The listing builds one solid part. Answer for the finished solid, in the listing's coordinates (mm). Face numbers are marked on the shaded views. A direction names the side the tool comes from. Give positions to 0.01 mm unless a question says otherwise; leave off trailing zeros. Loops run counter-clockwise (first coordinate to the right, second up) from the corner with the lowest first, then second, coordinate; pieces in that order, holes last. Notation, with made-up numbers: (44, 53) - (55, 53) arc R13 ccw to (55, 66) - close; hole circle Ø8 at (-26, 82). An arc over 180 degrees is marked (long way). Write item = value, one per line. Start each with the question number.
1) The part is cut by section D-D on z = 2.4. Write down the section's boundary in (x, y).
2) Flat-ended cylindrical pins translate along their axes: P1, Ø5.5, axis at x = 0, y = 0, coming from the +Z side; P2, Ø1.5, axis at x = -6.5, z = 2, coming from the +Y side. Find the tip coordinate at first contact, or state that the pin passes through.
3) The mould has two halves that part along Y. Classify the marked faces 4, 5, 6 and 7: +Y half, -Y half, draft (parallel to the pull), parting line (faces both ways), or undercut.
4) Consider probe 1 along Y at (x, z) = (0, 0.65) (3 decimals); probe 2 along Y at (x, z) = (7.5, 1.3); probe 3 along Y at (x, z) = (3.5, 1.3). Determine where each line is inside the solid, lowest interval first.
5) The part is cut by section C-C on x = -8. Write down the section's boundary in (y, z).
6) Which of the six approach directions +Z, -Z, +X, -X, +Y, -Y give full straight-line access (tool end or side, diameter ignored) to the marked faces 1, 2 and 3?
7) The part is cut by section A-A on y = 0. State how many separate pieces and enclosed holes the cut face has, plus the area to 3 significant figures.
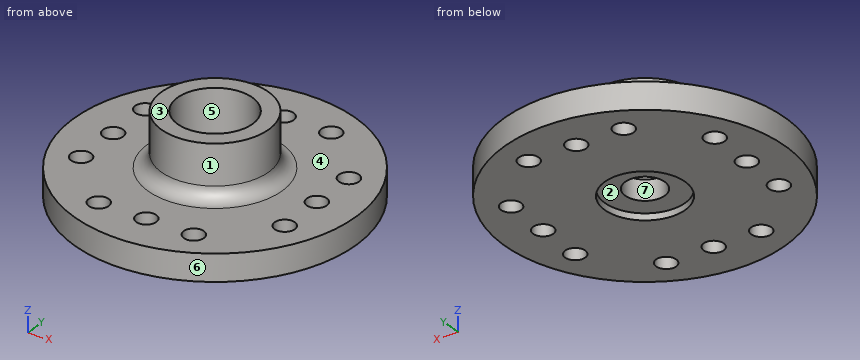
Autodesk Inventor part; units mm, degrees
ref_plane "YZ Plane" through (0, 0, 0) normal (1, 0, 0) x (0, 1, 0)
ref_plane "XZ Plane" through (0, 0, 0) normal (0, 1, 0) x (-1, 0, 0)
ref_plane "XY Plane" through (0, 0, 0) normal (0, 0, 1) x (1, 0, 0)
sketch "Boceto1" plane through (0, 0, 0) normal (0, 0, 1) x (1, 0, 0)
  circle A0 centre (0, 0) radius 10.5
  dimension "d0" = 21
extrude "Extrusión1" add sketch "Boceto1" along normal blind 2
sketch "Boceto2" plane through (0, 0, 2) normal (0, 0, 1) x (1, 0, 0)
  circle A0 centre (0, 0) radius 4
  dimension "d4" = 8
extrude "Extrusión2" add sketch "Boceto2" along normal blind 4
fillet "Empalme1" radius 1 1 edges at (-4, 0, 2)
sketch "Boceto3" plane through (0, 0, 6) normal (0, 0, 1) x (1, 0, 0)
  circle A0 centre (0, 0) radius 4
  circle A1 centre (0, 0) radius 2.8
  dimension "d8" = 5.6
extrude "Extrusión3" cut sketch "Boceto3" against normal blind 4 contours A1
sketch "Boceto4" plane through (0, 0, 2) normal (0, 0, 1) x (1, 0, 0)
  circle A0 centre (0, 0) radius 1.475
  dimension "d11" = 2.95
extrude "Extrusión4" cut sketch "Boceto4" against normal up to surface (2 mm away)
sketch "Boceto5" plane through (0, 0, 0) normal (0, 0, -1) x (-1, 0, 0)
  circle A0 centre (0, 0) radius 1.475
  circle A1 centre (0, 0) radius 3
  dimension "d14" = 6
extrude "Extrusión5" cut sketch "Boceto5" against normal blind 0.5
sketch "Boceto6" plane through (0, 0, 0) normal (0, 0, -1) x (-1, 0, 0)
  line L0 (11.1976, -7.5) -> (-9.8806, -7.5)
  circle A0 centre (0, -7.5) radius 0.75
  circle A1 centre (3.5, -7.5) radius 0.75
  circle A2 centre (-3.5, -7.5) radius 0.75
  circle A3 centre (7.5, 0) radius 0.75
  circle A4 centre (7.5, 3.5) radius 0.75
  circle A5 centre (7.5, -3.5) radius 0.75
  circle A6 centre (0, 7.5) radius 0.75
  circle A7 centre (-3.5, 7.5) radius 0.75
  circle A8 centre (3.5, 7.5) radius 0.75
  circle A9 centre (-7.5, 0) radius 0.75
  circle A10 centre (-7.5, -3.5) radius 0.75
  circle A11 centre (-7.5, 3.5) radius 0.75
  point P0 (0, 0)
  dimension "d17" = 7.5
  dimension "d18" = 1.5
  dimension "d19" = 3.5
  dimension "d20" = 3.5
  dimension "d23" = 360
extrude "Extrusión6" cut sketch "Boceto6" against normal through all
properties part number "horn"
Answer below:
q1.outline = circle Ø8.4 at (0, 0); hole circle Ø5.6 at (0, 0)
q2.P1 = 2
q2.P2 = 8.79
q3.face_4 = draft
q3.face_5 = undercut
q3.face_6 = parting line
q3.face_7 = undercut
q4.probe_1 = -10.5 to -8.25, -6.75 to -1.475, 1.475 to 6.75, 8.25 to 10.5
q4.probe_2 = -7.35 to -4.25, -2.75 to -0.75, 0.75 to 2.75, 4.25 to 7.35
q4.probe_3 = -9.9 to -8.25, -6.75 to 6.75, 8.25 to 9.9
q5.outline = (-6.8, 0) - (-4.06, 0) - (-4.06, 2) - (-6.8, 2) - close; (-2.94, 0) - (-0.56, 0) - (-0.56, 2) - (-2.94, 2) - close; (0.56, 0) - (2.94, 0) - (2.94, 2) - (0.56, 2) - close; (4.06, 0) - (6.8, 0) - (6.8, 2) - (4.06, 2) - close
q6.face_1 = +Z
q6.face_2 = -Z
q6.face_3 = +Z, +X, -X, +Y, -Y
q7.separate_pieces = 4
q7.enclosed_holes = 0
q7.area = 38.6 mm2
